```python
from build123d import *

# Parameters (mm, degrees)
SKETCH_1_R          = 1.5
SKETCH_1_R_2        = 1.1
EXTRUDE_1_DEPTH     = 6.5
SKETCH_2_R          = 4
SKETCH_2_R_2        = 1.1
EXTRUDE_2_DEPTH     = 1
EXTRUDE_3_DEPTH     = 9
SKETCH_4_R          = 2.5
EXTRUDE_4_DEPTH     = 10
SKETCH_5_R          = 4.5
CUT_EXTRUDE_1_DEPTH = 3
SKETCH_6_R          = 1.5
CUT_EXTRUDE_3_DEPTH = 6.5


with BuildPart() as part:
    # Эскиз1 → Бобышка-Вытянуть1 (new body)
    with BuildSketch(Plane(origin=(0, 0, 0), x_dir=(1, 0, 0), z_dir=(0, 1, 0))):
        with Locations(Location((0, 0, 0), (0, 0, 90))):
            Circle(SKETCH_1_R)
        with Locations(Location((0, 0, 0), (0, 0, 90))):
            Circle(SKETCH_1_R_2, mode=Mode.SUBTRACT)
    extrude(amount=EXTRUDE_1_DEPTH)

    # Эскиз2 → Бобышка-Вытянуть2 (add)
    with BuildSketch(Plane(origin=(0, 6.5, 0), x_dir=(1, 0, 0), z_dir=(0, 1, 0))):
        with Locations(Location((0, 0, 0), (0, 0, 270))):
            Circle(SKETCH_2_R)
        with Locations(Location((0, 0, 0), (0, 0, 90))):
            Circle(SKETCH_2_R_2, mode=Mode.SUBTRACT)
    extrude(amount=EXTRUDE_2_DEPTH)

    # Эскиз3 → Бобышка-Вытянуть3 (add)
    with BuildSketch(Plane(origin=(0, 7.5, 0), x_dir=(1, 0, 0), z_dir=(0, 1, 0))):
        with BuildLine():
            ThreePointArc((-3, 0), (-2.643382037, 1.418637165), (-1.658312395, 2.5))
            ThreePointArc((-1.658312395, 2.5), (0, 3), (1.658312395, 2.5))
            ThreePointArc((1.658312395, 2.5), (2.643382037, 1.418637165), (3, 0))
            Line((3, 0), (4, 0))
            ThreePointArc((4, 0), (0, 4), (-4, 0))
            Line((-4, 0), (-3, 0))
        make_face()
        with BuildLine():
            ThreePointArc((-1.658312395, -2.5), (-2.643382037, -1.418637165), (-3, 0))
            Line((-3, 0), (-4, 0))
            ThreePointArc((-4, 0), (0, -4), (4, 0))
            Line((4, 0), (3, 0))
            ThreePointArc((3, 0), (2.643382037, -1.418637165), (1.658312395, -2.5))
            ThreePointArc((1.658312395, -2.5), (0, -3), (-1.658312395, -2.5))
        make_face()
        with BuildLine():
            ThreePointArc((1.658312395, 2.5), (0, 3), (-1.658312395, 2.5))
            Line((-1.658312395, 2.5), (1.658312395, 2.5))
        make_face()
        with BuildLine():
            Line((1.658312395, -2.5), (-1.658312395, -2.5))
            ThreePointArc((-1.658312395, -2.5), (0, -3), (1.658312395, -2.5))
        make_face()
    extrude(amount=EXTRUDE_3_DEPTH)

    # Эскиз4 → Бобышка-Вытянуть4 (add)
    with BuildSketch(Plane.XZ.offset(-6.5)):
        with BuildLine():
            ThreePointArc((-0.727272727, 3.933328664), (4, 0), (-0.727272727, -3.933328664))
            Line((-0.727272727, -3.933328664), (9.909090909, -5.899992996))
            ThreePointArc((9.909090909, -5.899992996), (17, 0), (9.909090909, 5.899992996))
            Line((9.909090909, 5.899992996), (-0.727272727, 3.933328664))
        make_face()
        with Locations(Location((11, 0, 0), (0, 0, 270))):
            Circle(SKETCH_4_R, mode=Mode.SUBTRACT)
    extrude(amount=-EXTRUDE_4_DEPTH)

    # Эскиз5 → Вырез-Вытянуть1 (cut)
    with BuildSketch(Plane(origin=(0, 16.5, 0), x_dir=(1, 0, 0), z_dir=(0, 1, 0))):
        with Locations(Location((11, 0, 0), (0, 0, 270))):
            Circle(SKETCH_5_R)
    extrude(amount=-CUT_EXTRUDE_1_DEPTH, mode=Mode.SUBTRACT)

    # Эскиз6 → Вырез-Вытянуть3 (cut)
    with BuildSketch(Plane.XZ):
        Circle(SKETCH_6_R)
    extrude(amount=-CUT_EXTRUDE_3_DEPTH, mode=Mode.SUBTRACT)


solid = part.part
```
Part model, mm, in its own coordinate system. A direction names the side the tool comes from. Give positions to 0.01 mm unless a question says otherwise; leave off trailing zeros. Loops run counter-clockwise (first coordinate to the right, second up) from the corner with the lowest first, then second, coordinate; pieces in that order, holes last. Notation, with made-up numbers: M -4,45 L 55,45 A17 cw 55,77 Z; hole C 17,72.25 d7. An arc over 180 degrees is marked long. Return JSON: item names as keys, results as strings.
1) Saw through at B-B, the plane y = 15.5. List the corners of the cut face in (x, z), then the cut area to 3 significant figures.
Calculated:
{"outline": "M -0.73,-3.93 L 9.91,-5.9 A6 ccw long 9.91,5.9 L -0.73,3.93 A4 ccw Z; hole M -1.66,-2.5 L 1.66,-2.5 A3 ccw 1.66,2.5 L -1.66,2.5 A3 ccw Z; hole C 11,0 d9", "area": "104 mm2"}
2) Saw through at A-A, the plane x = 11. List the corners of the cut face in (y, z).
Calculated:
{"outline": "M 6.5,-6 L 16.5,-6 L 16.5,-4.5 L 13.5,-4.5 L 13.5,-2.5 L 6.5,-2.5 Z; M 6.5,2.5 L 13.5,2.5 L 13.5,4.5 L 16.5,4.5 L 16.5,6 L 6.5,6 Z"}
3) Saw through at C-C, the plane z = -0.25. List the corners of the cut face in (x, y), then the cut area to 3 significant figures.
Calculated:
{"outline": "M -3.99,6.5 L -1.07,6.5 L -1.07,7.5 L -2.99,7.5 L -2.99,16.5 L -3.99,16.5 Z; M 1.07,6.5 L 8.51,6.5 L 8.51,13.5 L 6.51,13.5 L 6.51,16.5 L 2.99,16.5 L 2.99,7.5 L 1.07,7.5 Z; M 13.49,6.5 L 16.99,6.5 L 16.99,16.5 L 15.49,16.5 L 15.49,13.5 L 13.49,13.5 Z", "area": "92.1 mm2"}
4) 3-axis set-ups, long thin cutter, end or side, ignore diameter. For faces 1 (the face through (4.5, 11.4, -4.9)), 2 (the face through (9, 13.5, 2)): which of +Z, -Z, +X, -X, +Y, -Y reach the whole face in a straight line?
Calculated:
{"face 1": "-Z, -X, +Y, -Y", "face 2": "+Y"}
5) Saw through at D-D, the plane y = 13. List the corners of the cut face in (x, z).
Calculated:
{"outline": "M -0.73,-3.93 L 9.91,-5.9 A6 ccw long 9.91,5.9 L -0.73,3.93 A4 ccw Z; hole M -1.66,-2.5 L 1.66,-2.5 A3 ccw 1.66,2.5 L -1.66,2.5 A3 ccw Z; hole C 11,0 d5"}
6) Drill centre lines: line 1 (X direction, y = 6.8, z = 0); line 2 (X direction, y = 13.75, z = 1); line 3 (Y direction, x = 10.5, z = -3). Where is each one in solid material? Low to high.
Calculated:
{"line 1": "x = -4 to -1.1, 1.1 to 8.5, 13.5 to 17", "line 2": "x = -3.87 to -2.83, 2.83 to 6.61, 15.39 to 16.92", "line 3": "y = 6.5 to 13.5"}
7) Flat gauge pins, fed straight in: pin 1 Ø2.5 at (x, z) = (0.5, 0) entering from +Y; pin 2 Ø1 at (x, y) = (-0.5, 11.5) entering from +Z; pin 3 Ø1 at (x, z) = (11, 0) entering from -Y; pin 4 Ø3 at (x, y) = (4.5, 9) entering from +Z. Where does each tip first touch, or does it go through?
Calculated:
{"pin 1": "stops at y = 7.5", "pin 2": "stops at z = 4.07", "pin 3": "passes through", "pin 4": "stops at z = 5.18"}
